Input: part model. Units: mm. Frame: model coordinates. A direction names the side the tool comes from. Give positions to 0.01 mm unless a question says otherwise; leave off trailing zeros. Loops run counter-clockwise (first coordinate to the right, second up) from the corner with the lowest first, then second, coordinate; pieces in that order, holes last. Notation, with made-up numbers: (71.25, 5.25) -> (75.25, 5.25) arc R13 ccw to (75.25, 20.25) -> close; hole circle Ø6 at (8, -14.5). An arc over 180 degrees is marked (long way). Use CSV: the item, a comma, the result in double quotes.
```python
from build123d import *

# Parameters (mm, degrees)
F0_R     = 5
F0_R_2   = 1.5
F1_DEPTH = 7.25
F2_R     = 12.5
F3_DEPTH = 1
F4_R     = 2
F5_DEPTH = 5
F6_R     = 2


with BuildPart() as f1:
    # F0 (on Front) → F1 (new body)
    with BuildSketch(Plane.XZ):
        Circle(F0_R)
        Circle(F0_R_2, mode=Mode.SUBTRACT)
    extrude(amount=F1_DEPTH)

    # F2 (on face) → F3 (join)
    with BuildSketch(Plane.XZ.offset(7.25)):
        Circle(F2_R)
    extrude(amount=F3_DEPTH)

    # F4 (on face) → F5 (join)
    with BuildSketch(Plane.XZ.offset(8.25)):
        Circle(F4_R)
    extrude(amount=F5_DEPTH)

    # F6
    f6_edges = [f1.edges().sort_by_distance(p)[0] for p in [
        (-2, -13.25, 0),
    ]]
    fillet(f6_edges, radius=F6_R)


solid = f1.part
```
1) Section query B-B (x = 0). Return loops of the section in (y, z).
From the geometry:
outline,"(-11.25, -2) -> (-8.25, -2) -> (-8.25, -12.5) -> (-7.25, -12.5) -> (-7.25, -5) -> (0, -5) -> (0, -1.5) -> (-7.25, -1.5) -> (-7.25, 1.5) -> (0, 1.5) -> (0, 5) -> (-7.25, 5) -> (-7.25, 12.5) -> (-8.25, 12.5) -> (-8.25, 2) -> (-11.25, 2) arc R2 ccw to start"
2) Reachability of faces 4 (the flat face through (-1.2, 0, 1.2)), 5 (the cylindrical face through (-1.08, -3.57, -4.88)) from +Z, -Z, +X, -X, +Y, -Y: full face, straight path, thin tool, end or side. Return the list, or none.
From the geometry:
face 4,"+Z, -Z, +X, -X, +Y"
face 5,"+Y"
3) Ray query, line 1 (Z direction, x = 0, y = -4.5); line 2 (Y direction, x = -3.75, z = 6.25); line 3 (Z direction, x = -1, y = -5.25). Return the intervals inside material, ascending.
From the geometry:
line 1,"z = -5 to -1.5, 1.5 to 5"
line 2,"y = -8.25 to -7.25"
line 3,"z = -4.9 to -1.12, 1.12 to 4.9"
4) Section query D-D (z = -2.5). Return loops of the section in (x, y).
From the geometry:
outline,"(-12.25, -8.25) -> (12.25, -8.25) -> (12.25, -7.25) -> (4.33, -7.25) -> (4.33, 0) -> (-4.33, 0) -> (-4.33, -7.25) -> (-12.25, -7.25) -> close"
5) Mould query, pull axis X, two halves, no side actions, for faces 1 (the flat face through (-0.2, -7.25, -5.4)), 2 (the cylindrical face through (0, -10, -2)), 3 (the flat face through (0, -7.25, 0)). Classes: pulls with the +X half, pulls with the -X half, needs draft (parallel to the pull), parting line crosses it, or undercut.
From the geometry:
face 1,"needs draft"
face 2,"parting line crosses it"
face 3,"undercut"
6) Contact query for flat-ended pins moving along their axis: pin 1 (1.5 mm diameter, centred on x = 0.5, z = -0.5, fed in from +Y); pin 2 (3 mm diameter, centred on y = -10.5, z = -2.5, fed in from +X); pin 3 (7.5 mm diameter, centred on x = 5, z = -6, fed in from -Y). Output: stop coordinate, or through.
From the geometry:
pin 1,"stops at y = -7.25"
pin 2,"stops at x = 1.73"
pin 3,"stops at y = -8.25"
7) Section query A-A (z = 0). Return loops of the section in (x, y).
From the geometry:
outline,"(-12.5, -8.25) -> (-2, -8.25) -> (-2, -11.25) arc R2 ccw to (2, -11.25) -> (2, -8.25) -> (12.5, -8.25) -> (12.5, -7.25) -> (5, -7.25) -> (5, 0) -> (1.5, 0) -> (1.5, -7.25) -> (-1.5, -7.25) -> (-1.5, 0) -> (-5, 0) -> (-5, -7.25) -> (-12.5, -7.25) -> close"
8) Section query C-C (y = -2.5). Return loops of the section in (x, z).
From the geometry:
outline,"circle Ø10 at (0, 0); hole circle Ø3 at (0, 0)"
